Here's the drawing with two shaded views (mm, measured from the low corner). I have some questions. A direction names the side the tool comes from. Give positions to 0.01 mm unless a question says otherwise; leave off trailing zeros. Write each loop counter-clockwise with the first axis right and the second up, starting at its lowest first coordinate (ties: lowest second). Pieces come first, ordered by that corner, then holes. Notation, with made-up numbers: (61.5, 60) -> (77.5, 60) arc R9 cw to (77.5, 75) -> close; hole circle Ø11 at (-27.75, 41). An arc over 180 degrees is marked (long way). One line per item, written item: value.
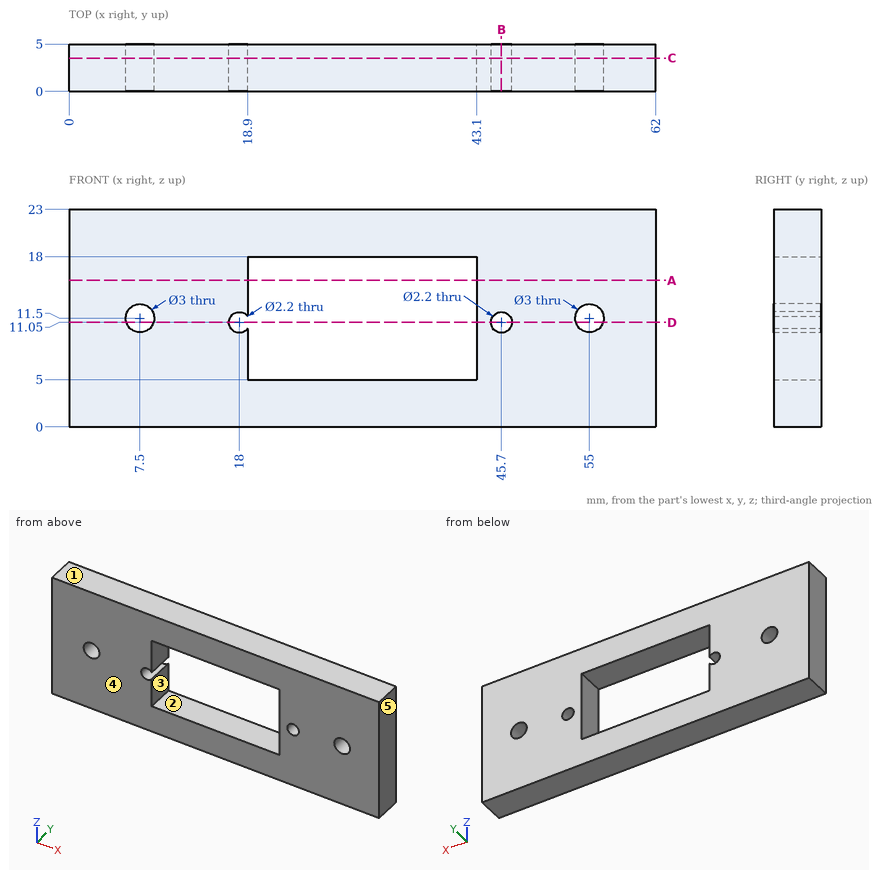
1) If we section it at A-A (z = 15.5): Write out the boundary of the cut face in (x, y), and give its area (3 significant figures).
Answer list:
outline: (0, 0) -> (18.9, 0) -> (18.9, 5) -> (0, 5) -> close; (43.1, 0) -> (62, 0) -> (62, 5) -> (43.1, 5) -> close
area: 189 mm^2
2) I need wall thicknesses on L1, parallel to Z at x = 33, y = 4.15; L2, parallel to X at y = 2.4, z = 11.05; L3, parallel to X at y = 3.25, z = 11.5. Which ranges of each line are inside material? Lowest first, please.
Answer list:
L1: z = 0 to 5, 18 to 23
L2: x = 0 to 6.07, 8.93 to 16.9, 43.1 to 44.6, 46.8 to 53.57, 56.43 to 62
L3: x = 0 to 6, 9 to 17, 43.1 to 44.7, 46.7 to 53.5, 56.5 to 62
3) We'd pull the mould along X, two halves only. Please class the marked faces 3, 4 and 5: released by +X, released by -X, zero draft, split by the parting line, or undercut.
Answer list:
face 3: undercut
face 4: zero draft
face 5: released by +X
4) For the marked faces 1 and 2, which set-ups out of +Z, -Z, +X, -X, +Y, -Y let a thin tool reach every point of the face, with its end or its side?
Answer list:
face 1: +Z, +X, -X, +Y, -Y
face 2: +Y, -Y
5) If we section it at B-B (x = 45.7): Write out the boundary of the cut face in (y, z).
Answer list:
outline: (0, 0) -> (5, 0) -> (5, 9.95) -> (0, 9.95) -> close; (0, 12.15) -> (5, 12.15) -> (5, 23) -> (0, 23) -> close
6) If we section it at C-C (y = 3.5): Write out the boundary of the cut face in (x, z), and give its area (3 significant figures).
Answer list:
outline: (0, 0) -> (62, 0) -> (62, 23) -> (0, 23) -> close; hole circle Ø3 at (7.5, 11.5); hole (18.9, 5) -> (43.1, 5) -> (43.1, 18) -> (18.9, 18) -> (18.9, 11.68) arc R1.1 ccw (long way) to (18.9, 10.42) -> close; hole circle Ø2.2 at (45.7, 11.05); hole circle Ø3 at (55, 11.5)
area: 1,090 mm^2
7) If we section it at D-D (z = 11.05): Write out the boundary of the cut face in (x, y), and give its area (3 significant figures).
Answer list:
outline: (0, 0) -> (6.07, 0) -> (6.07, 5) -> (0, 5) -> close; (8.93, 0) -> (16.9, 0) -> (16.9, 5) -> (8.93, 5) -> close; (43.1, 0) -> (44.6, 0) -> (44.6, 5) -> (43.1, 5) -> close; (46.8, 0) -> (53.57, 0) -> (53.57, 5) -> (46.8, 5) -> close; (56.43, 0) -> (62, 0) -> (62, 5) -> (56.43, 5) -> close
area: 139 mm^2
